Check sheet for the modelled part. Datum: model origin and axes. Units: mm. Face numbers are marked on the shaded views. A direction names the side the tool comes from. Give positions to 0.01 mm unless a question says otherwise; leave off trailing zeros. Loops run counter-clockwise (first coordinate to the right, second up) from the corner with the lowest first, then second, coordinate; pieces in that order, holes last. Notation, with made-up numbers: (-39, 24) -> (-5, 24) arc R14 cw to (-5, 39) -> close; hole circle Ø9 at (35, 44.5). An arc over 180 degrees is marked (long way). Write each question's results on one line, items separated by ' | '. Start each with the question number.
Item 1: Mould release check, pull along X, two halves, no side actions. Record for the marked faces 1, 2 and 3: pulls with the +X half, pulls with the -X half, needs draft (parallel to the pull), parting line crosses it, or undercut.
Item 2: Cross-section at C-C on y = 25.5. Enter the section's corners in (x, z), then the cut area to 3 significant figures.
Item 3: Scan lines: line 1 along Y through (x, z) = (-36, 0.65); line 2 along Y through (x, z) = (-39, 1.3); line 3 along X through (y, z) = (25.25, 1.35). Record each from-to range of solid material in increasing order.
Item 4: Cross-section at D-D on x = -30. Enter the section's corners in (y, z).
Item 5: Cross-section at B-B on x = -12.5. Enter the section's corners in (y, z), then the cut area to 3 significant figures.
Item 6: Cross-section at A-A on y = 28.75. Enter the section's corners in (x, z), then the cut area to 3 significant figures.
Item 7: Access from +Z, -Z, +X, -X, +Y, -Y to the whole of each face (thin tool, end or side, straight path). Record for the marked faces 4, 5, 6 and 7.
Item 8: Gauge pin test, flat ends, axial feed: pin 1 Ø0.9 at (x, z) = (-39, 2) entering from -Y; pin 2 Ø0.9 at (y, z) = (20.5, 1) entering from -X; pin 3 Ø0.9 at (y, z) = (31, 1) entering from +X. Record the tip position at first contact, or that the pin passes through.
from build123d import *

# Parameters (mm, degrees)
SKETCH1_R      = 2.2795
SKETCH1_W      = 3.88
SKETCH1_H      = 3.007
EXTRUDE1_DEPTH = 3.1


with BuildPart() as part:
    # Sketch1 → Extrude1 (new body)
    with BuildSketch(Plane.XY):
        with BuildLine():
            Line((-41.027382287, 34.508489293), (-10.498924525, 34.508489293))
            Line((-10.498924525, 34.508489293), (-10.513157114, 32.461989293))
            Line((-10.513157114, 32.461989293), (-18.030657114, 32.461989293))
            Line((-18.030657114, 32.461989293), (-18.030657114, 29.454989293))
            Line((-18.030657114, 29.454989293), (-10.513157114, 29.454989293))
            Line((-10.513157114, 29.454989293), (-10.513157114, 26.058489293))
            ThreePointArc((-10.513157114, 26.058489293), (-10.83664158, 24.508533678), (-11.7530861, 23.217358224))
            Line((-11.7530861, 23.217358224), (-23.1280861, 12.667358224))
            ThreePointArc((-23.1280861, 12.667358224), (-25.763157114, 11.633489293), (-28.398228128, 12.667358224))
            Line((-28.398228128, 12.667358224), (-39.773228128, 23.217358224))
            ThreePointArc((-39.773228128, 23.217358224), (-40.689672648, 24.508533678), (-41.013157114, 26.058489293))
            Line((-41.013157114, 26.058489293), (-41.013157114, 29.454989293))
            Line((-41.013157114, 29.454989293), (-33.495657114, 29.454989293))
            Line((-33.495657114, 29.454989293), (-33.495657114, 32.461989293))
            Line((-33.495657114, 32.461989293), (-41.013157114, 32.461989293))
            Line((-41.013157114, 32.461989293), (-41.027382287, 34.508489293))
        make_face()
        with Locations(Location((-14.388157114, 26.058489293, 0), (0, 0, 180))):
            Circle(SKETCH1_R, mode=Mode.SUBTRACT)
        with Locations(Location((-37.138157114, 26.058489293, 0), (0, 0, 180))):
            Circle(SKETCH1_R, mode=Mode.SUBTRACT)
        with Locations(Location((-25.763157114, 15.508489293, 0), (0, 0, 180))):
            Circle(SKETCH1_R, mode=Mode.SUBTRACT)
        with BuildLine():
            Line((-33.76750302, 22.568552775), (-31.002944054, 20.130132194))
            Line((-31.002944054, 20.130132194), (-30.638157114, 20.130132194))
            ThreePointArc((-30.638157114, 20.130132194), (-29.931050333, 20.423025412), (-29.638157114, 21.130132194))
            Line((-29.638157114, 21.130132194), (-29.638157114, 22.458489293))
            ThreePointArc((-29.638157114, 22.458489293), (-29.345263895, 23.165596075), (-28.638157114, 23.458489293))
            Line((-28.638157114, 23.458489293), (-22.889213944, 23.458489293))
            ThreePointArc((-22.889213944, 23.458489293), (-22.182388419, 23.165877219), (-21.889214261, 22.459284647))
            Line((-21.889214261, 22.459284647), (-21.888157114, 21.130132194))
            ThreePointArc((-21.888157114, 21.130132194), (-21.595263895, 20.423025412), (-20.888157114, 20.130132194))
            Line((-20.888157114, 20.130132194), (-20.523370174, 20.130132194))
            Line((-20.523370174, 20.130132194), (-17.758811208, 22.568552775))
            ThreePointArc((-17.758811208, 22.568552775), (-17.428169762, 23.19327051), (-17.593190704, 23.880558008))
            ThreePointArc((-17.593190704, 23.880558008), (-17.720651816, 24.081090988), (-17.835582513, 24.289059126))
            ThreePointArc((-17.835582513, 24.289059126), (-18.600140603, 25.542598068), (-19.540017718, 26.670667198))
            Line((-19.540017718, 26.670667198), (-21.890008982, 29.103277241))
            ThreePointArc((-21.890008982, 29.103277241), (-22.218575416, 29.329029338), (-22.609223629, 29.408489293))
            Line((-22.609223629, 29.408489293), (-28.917090599, 29.408489293))
            ThreePointArc((-28.917090599, 29.408489293), (-29.307738812, 29.329029338), (-29.636305246, 29.103277241))
            Line((-29.636305246, 29.103277241), (-31.98629651, 26.670667198))
            ThreePointArc((-31.98629651, 26.670667198), (-32.926173625, 25.542598068), (-33.690731715, 24.289059126))
            ThreePointArc((-33.690731715, 24.289059126), (-33.805662411, 24.081090988), (-33.933123524, 23.880558008))
            ThreePointArc((-33.933123524, 23.880558008), (-34.098144466, 23.19327051), (-33.76750302, 22.568552775))
        make_face(mode=Mode.SUBTRACT)
        with Locations((-25.763157114, 20.408489293)):
            Rectangle(SKETCH1_W, SKETCH1_H, mode=Mode.SUBTRACT)
    extrude(amount=EXTRUDE1_DEPTH)


solid = part.part
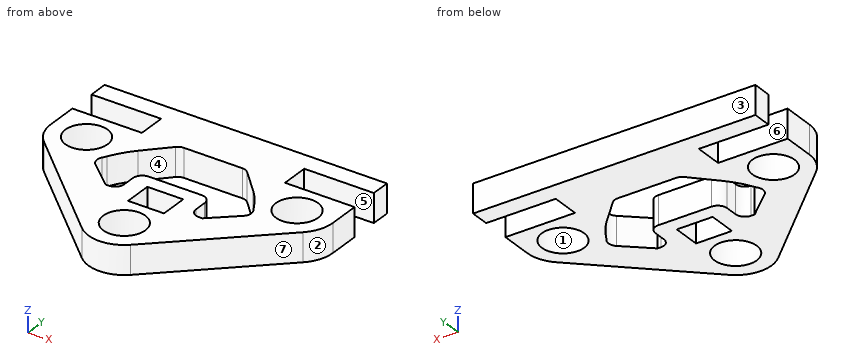
Answer sheet:
1) face 1: undercut | face 2: pulls with the +X half | face 3: needs draft
2) outline: (-40.97, 0) -> (-39.35, 0) -> (-39.35, 3.1) -> (-40.97, 3.1) -> close; (-34.93, 0) -> (-32.96, 0) -> (-32.96, 3.1) -> (-34.93, 3.1) -> close; (-18.57, 0) -> (-16.6, 0) -> (-16.6, 3.1) -> (-18.57, 3.1) -> close; (-12.18, 0) -> (-10.55, 0) -> (-10.55, 3.1) -> (-12.18, 3.1) -> close | area: 22.3 mm²
3) line 1: y = 19.72 to 24.08, 28.03 to 29.45, 32.46 to 34.51 | line 2: y = 22.5 to 24.74, 27.37 to 29.45, 32.46 to 34.51 | line 3: x = -40.93 to -39.27, -35.01 to -33.13, -18.4 to -16.52, -12.26 to -10.6
4) outline: (14.15, 0) -> (20.36, 0) -> (20.36, 3.1) -> (14.15, 3.1) -> close; (28.73, 0) -> (34.51, 0) -> (34.51, 3.1) -> (28.73, 3.1) -> close
5) outline: (22.52, 0) -> (24.78, 0) -> (24.78, 3.1) -> (22.52, 3.1) -> close; (27.34, 0) -> (29.45, 0) -> (29.45, 3.1) -> (27.34, 3.1) -> close; (32.46, 0) -> (34.51, 0) -> (34.51, 3.1) -> (32.46, 3.1) -> close | area: 19.9 mm²
6) outline: (-41.01, 0) -> (-29.98, 0) -> (-29.98, 3.1) -> (-41.01, 3.1) -> close; (-21.55, 0) -> (-10.51, 0) -> (-10.51, 3.1) -> (-21.55, 3.1) -> close | area: 68.4 mm²
7) face 4: +Z, -Z | face 5: +Z, -Z, +X | face 6: +Z, -Z, -X | face 7: +Z, -Z, +X, -Y
8) pin 1: stops at y = 22.08 | pin 2: stops at x = -37.33 | pin 3: stops at x = -18.03
